Autodesk Inventor part; units mm, degrees
ref_plane "YZ Plane" through (0, 0, 0) normal (1, 0, 0) x (0, 1, 0)
ref_plane "XZ Plane" through (0, 0, 0) normal (0, 1, 0) x (-1, 0, 0)
ref_plane "XY Plane" through (0, 0, 0) normal (0, 0, 1) x (1, 0, 0)
sketch "スケッチ1" plane through (0, 0, 0) normal (0, 1, 0) x (-1, 0, 0)
  line L0 (26, 0) -> (0, 0)
  line L1 (0, 0) -> (0, -33)
  line L2 (0, -33) -> (26, -33)
  line L3 (26, -33) -> (26, 0)
  line L4 (26, -9) -> (0, -9)
  line L5 (0, -9) -> (0, -33)
  line L6 (0, -33) -> (26, -33)
  line L7 (26, -33) -> (26, -9)
  circle A0 centre (13, -9) radius 13
  circle A1 centre (13, -9) radius 6.25
  circle A2 centre (13, -9) radius 27.2947
  circle A3 centre (13, -9) radius 32.2947
  circle A4 centre (13, -9) radius 15
  line L8 (28, -9) -> (-2, -9)
  line L9 (-2, -9) -> (-2, -35)
  line L10 (-2, -35) -> (28, -35)
  line L11 (28, -35) -> (28, -9)
  line L12 (23.198, 2) -> (2.802, 2)
  line L13 (13, -9) -> (40.968, -25.1473)
  line L14 (13, -9) -> (-14.968, -25.1473)
  point P0 (22.3808, 0)
  point P1 (3.6192, 0)
  point P2 (0, -9)
  point P3 (-17.3636, 2)
  point P4 (43.3636, 2)
  point P5 (25, 0)
  point P6 (26, -1.5167)
  point P7 (0, -1.5167)
  point P8 (1, 0)
  point P9 (21.3066, -35)
  point P10 (4.6934, -35)
  point P11 (0, -16.4833)
  point P12 (26, -16.4833)
  point P13 (0, -9)
  point P14 (26, -9)
  point P15 (28, -17.6603)
  point P16 (-2, -17.6603)
  point P17 (28, -31.8035)
  point P18 (-2, -31.8035)
  dimension "d0" = 26
  dimension "d1" = 33
  dimension "d2" = 24
  dimension "d3" = 12.5
  dimension "d6" = 5
  dimension "d7" = 2
  dimension "d8" = 2
  dimension "d9" = 2
  dimension "d16" = 60
  dimension "d17" = 60
extrude "押し出し1" add sketch "スケッチ1" against normal blind 1.5 contours A0 L4 A1 L0 | A0 L13 A1 L4 | L3 A4 L13 A0 | L3 L13 A4 | L13 A4 L14 A0 | A0 L14 A1 L13 | A0 L14 A4 L1 | L4 A1 L14 A0 | L3 L2 L1 L14 A4 L13 | A4 L14 L1
extrude "押し出し2" add sketch "スケッチ1" against normal blind 27.5 contours A4 L3 A0 L0 | L0 A0 L12 A4 | A4 L8 L3 | L0 A0 L12 | L8 A4 L3 | L11 L13 L3 A4 | A0 L1 A4 L0 | L0 A4 L12 A0 | L11 A2 L3 L13 | L8 A4 L1 | L1 A4 L8 | L1 L14 L9 A4 | A2 L10 L2 | L1 A2 L9 L14
extrude "押し出し3" add sketch "スケッチ1" against normal blind 22.5 contours L13 A2 L11 | L11 L10 A2 | A2 L13 A3 L14 L9 L10 L11 | L9 A2 L14 | A2 L10 L9 | A2 L10
extrude "押し出し4" cut sketch "スケッチ1" against normal blind 17.5 contours L13 A2 L11 | L11 L10 A2 | A2 L13 A3 L14 L9 L10 L11 | L9 A2 L14 | A2 L10 L9 | A2 L10
sketch "スケッチ2" plane through (2, -27.5, -9) normal (1, 0, 0) x (0, 0, -1)
  line L0 (17.5, 16.8) -> (4, 16.8)
  line L1 (4, 16.8) -> (4, 18.5)
  line L2 (4, 18.5) -> (0, 18.5)
  line L3 (0, 12.5) -> (0, 18.5)
  line L4 (0, 12.5) -> (21, 12.5)
  line L5 (21, 12.5) -> (21, 18.5)
  line L6 (21, 18.5) -> (17.5, 18.5)
  line L7 (17.5, 18.5) -> (17.5, 16.8)
  line L8 (4, 22.9122) -> (17.5, 22.9122)
  line L9 (17.5, 22.9122) -> (17.5, 19)
  line L10 (17.5, 19) -> (21, 19)
  line L11 (21, 19) -> (21, 26)
  line L12 (21, 26) -> (0, 26)
  line L13 (0, 19) -> (0, 26)
  line L14 (0, 19) -> (4, 19)
  line L15 (4, 19) -> (4, 22.9122)
  line L16 (4, 16.8) -> (17.5, 16.8)
  line L17 (17.5, 16.8) -> (17.5, 22.9122)
  line L18 (17.5, 22.9122) -> (4, 22.9122)
  line L19 (4, 22.9122) -> (4, 16.8)
  point P0 (-9, 27.5)
  point P1 (4, 19)
  point P2 (4, 18.5)
extrude "押し出し5" cut sketch "スケッチ2" against normal up to surface (2 mm away) contours L0 L1 L19 L15 L8 L9 L17 L7
sketch "スケッチ3" plane through (0, 0, 0) normal (0, 1, 0) x (1, 0, 0)
  circle A0 centre (-2.5, 30) radius 0.85
  circle A1 centre (-23.5, 30) radius 0.85
  circle A2 centre (-23.5, 9) radius 0.85
  circle A3 centre (-2.5, 9) radius 0.85
  point P0 (0, 0)
extrude "押し出し6" cut sketch "スケッチ3" against normal blind 10
equation "\"d17\" = d16"
properties part number "waist"
Here's how the part is built. I have some questions about the finished solid (model axes, mm). A direction names the side the tool comes from. Give positions to 0.01 mm unless a question says otherwise; leave off trailing zeros. Write each loop counter-clockwise with the first axis right and the second up, starting at its lowest first coordinate (ties: lowest second). Pieces come first, ordered by that corner, then holes. Notation, with made-up numbers: M 3,-30 L 32,-30 A33 ccw 32,5 Z; hole C -18,85 d5. An arc over 180 degrees is marked long. Put each result on its own line as item: value. Start each with the question number.
Item 1: If we section it at A-A, the plane x = -13: Write out the boundary of the cut face in (y, z).
Item 2: I need wall thicknesses on L1, parallel to X at y = -0.35, z = -9; L2, parallel to X at y = -2.75, z = -15; L3, parallel to X at y = -0.9, z = -30. Which ranges of each line are inside material? Lowest first, please. Write a range as from..to.
Item 3: If we section it at B-B, the plane y = -3: Write out the boundary of the cut face in (x, z), then the cut area to 3 significant figures.
Item 4: Will these pins go through, and if not, where does the flat tip stop? pin 1 (2 mm diameter, centred on x = -2.5, z = -9, fed in from -Y); pin 2 (6 mm diameter, centred on y = -4, z = -4, fed in from -X); pin 3 (1.5 mm diameter, centred on x = -12, y = -24.5, fed in from -Z).
Item 5: On a 3-axis mill with a long thin cutter (end or side, diameter ignored), from which of +Z, -Z, +X, -X, +Y, -Y can I reach the whole of each face in a straight line? I mean faces 5 (the cylindrical face through (1.027, -24.965, -32.415)), 6 (the flat face through (-13, -14, -33)), 7 (the flat face through (-13, -22.5, -36)). Say none if no direction works.
Item 6: If we section it at C-C, the plane z = -23: Write out the boundary of the cut face in (x, y), then the cut area to 3 significant figures.
Item 7: If we section it at D-D, the plane x = -27: Write out the boundary of the cut face in (y, z), then the cut area to 3 significant figures.
Item 8: Thinking about a two-plate mould opening in X: for faces 1 (the cylindrical face through (-24.35, -0.74, -9.04)), 2 (the flat face through (-13, -17.5, -36)), 3 (the cylindrical face through (-24.1, -0.7, -30.6)), 4 (the cylindrical face through (-26.782, -13.558, -3.078)), which applies, +X half, -X half, draft (parallel to the pull), parting line (faces both ways), or undercut?
Values:
1. outline: M -27.5,-35 L -22.5,-35 L -22.5,-41.29 L -17.5,-41.29 L -17.5,-35 L 0,-35 L 0,-15.25 L -1.5,-15.25 L -1.5,-33 L -27.5,-33 Z; M -27.5,0 L -1.5,0 L -1.5,-2.75 L 0,-2.75 L 0,2 L -27.5,2 Z
2. L1: -28..-24.35, -22.65..-19.25, -6.75..-3.35, -1.65..2
2. L2: -28..-26, 0..2
2. L3: -28..-24.35, -22.65..-3.35, -1.65..2
3. outline: M -28,-31.8 A27.29 ccw -21.31,-35 L -4.69,-35 A27.29 ccw 2,-31.8 L 2,-9 A15 ccw -2.8,2 L -23.2,2 A15 ccw -28,-9 Z; hole M -26,-33 L 0,-33 L 0,-9 A13 ccw -3.62,0 L -22.38,0 A13 ccw -26,-9 Z
3. area: 221 mm²
4. pin 1: y = -1.5
4. pin 2: x = -27.87
4. pin 3: z = -35
5. face 5: -Z, +X, -Y
5. face 6: -Y
5. face 7: -Z, -Y
6. outline: M -37.25,-22.5 L -28,-22.5 L -28,-27.5 L -26,-27.5 L -26,-1.5 L 0,-1.5 L 0,-4.59 L 2,-4.59 L 2,0 L -28,0 L -28,-17.5 L -37.25,-17.5 Z; M 0,-27.5 L 2,-27.5 L 2,-22.5 L 11.25,-22.5 L 11.25,-17.5 L 2,-17.5 L 2,-10.7 L 0,-10.7 Z
6. area: 229 mm²
7. outline: M -27.5,-32.43 L -22.5,-32.43 L -22.5,-38.1 L -17.5,-38.1 L -17.5,-32.43 L 0,-32.43 L 0,-3.61 L -27.5,-3.61 Z
7. area: 821 mm²
8. face 1: undercut
8. face 2: draft
8. face 3: undercut
8. face 4: -X half
